Design review of the part built by this model. Coordinates are the model's own, in mm. Coordinates: 2 decimals unless noted, no trailing zeros. Write each loop counter-clockwise with the first axis right and the second up, starting at its lowest first coordinate (ties: lowest second). Pieces come first, ordered by that corner, then holes.
Q1. Take a section at A-A (z = 11.5). Give the boundary of the cut face in (x, y) (3 decimals), and give its area (3 significant figures).
Q2. Mouldability with a two-part tool opening along X and no side actions: class faces 1 (the cylindrical face through (30.229, 1.493, -18.726)), 2 (the cylindrical face through (-16.854, 1.479, -12.63)), 3 (the flat face through (3, 3, 2)) as pulls with the +X half, pulls with the -X half, needs draft (parallel to the pull), parting line crosses it, or undercut.
Q3. For probe 1 along X at (y, z) = (1.8, 11.5) (3 decimals); probe 2 along X at (y, z) = (1.7, -12.5) (3 decimals); probe 3 along X at (y, z) = (2.3, 11.5) (3 decimals), list the stretches that pass through material, from the lowest coordinate up.
Q4. Take a section at B-B (z = -12.5). Give the boundary of the cut face in (x, y) (3 decimals).
```python
from build123d import *

# Parameters (mm, degrees)
SKETCH1_R           = 1
BOSS_EXTRUDE1_DEPTH = 3
FILLET1_R           = 1


with BuildPart() as part:
    # Sketch1 → Boss-Extrude1 (new body)
    with BuildSketch(Plane(origin=(0, 0, 0), x_dir=(-1, 0, 0), z_dir=(0, 1, 0))):
        with BuildLine():
            Line((-31.655, 18.23), (-31.655, -15.23))
            ThreePointArc((-31.655, -15.23), (-30.190533906, -18.765533906), (-26.655, -20.23))
            Line((-26.655, -20.23), (20.655, -20.23))
            ThreePointArc((20.655, -20.23), (24.190533906, -18.765533906), (25.655, -15.23))
            Line((25.655, -15.23), (25.655, 18.23))
            ThreePointArc((25.655, 18.23), (24.190533906, 21.765533906), (20.655, 23.23))
            Line((20.655, 23.23), (-26.655, 23.23))
            ThreePointArc((-26.655, 23.23), (-30.190533906, 21.765533906), (-31.655, 18.23))
        make_face()
        with Locations(Location((-18.155, 11.5, 0), (0, 0, 90))):
            Circle(SKETCH1_R, mode=Mode.SUBTRACT)
        with Locations(Location((17.845, 11.5, 0), (0, 0, 90))):
            Circle(SKETCH1_R, mode=Mode.SUBTRACT)
        with Locations(Location((17.845, -12.5, 0), (0, 0, 90))):
            Circle(SKETCH1_R, mode=Mode.SUBTRACT)
    extrude(amount=BOSS_EXTRUDE1_DEPTH)

    # Fillet1
    fillet1_edges = [part.edges().sort_by_distance(p)[0] for p in [
        (30.190533906, 3, -18.765533906),
        (31.655, 0, 1.5),
        (30.190533906, 0, 21.765533906),
        (3, 3, -20.23),
        (-24.190533906, 3, -18.765533906),
        (-25.655, 3, 1.5),
        (-24.190533906, 3, 21.765533906),
        (3, 3, 23.23),
        (30.190533906, 3, 21.765533906),
        (31.655, 3, 1.5),
        (3, 0, 23.23),
        (-24.190533906, 0, 21.765533906),
        (-25.655, 0, 1.5),
        (-24.190533906, 0, -18.765533906),
        (3, 0, -20.23),
        (30.190533906, 0, -18.765533906),
    ]]
    fillet(fillet1_edges, radius=FILLET1_R)


solid = part.part
```
Response:
1. outline: (-25.655, 1) arc R1 ccw to (-24.655, 0) - (-18.845, 0) - (-18.845, 3) - (-24.655, 3) arc R1 ccw to (-25.655, 2) - close; (-16.845, 0) - (17.155, 0) - (17.155, 3) - (-16.845, 3) - close; (19.155, 0) - (30.655, 0) arc R1 ccw to (31.655, 1) - (31.655, 2) arc R1 ccw to (30.655, 3) - (19.155, 3) - close
1. area: 159 mm2
2. face 1: pulls with the +X half
2. face 2: undercut
2. face 3: needs draft
3. probe 1: x = -25.655 to -18.845, -16.845 to 17.155, 19.155 to 31.655
3. probe 2: x = -25.655 to -18.845, -16.845 to 31.655
3. probe 3: x = -25.609 to -18.845, -16.845 to 17.155, 19.155 to 31.609
4. outline: (-25.655, 1) arc R1 ccw to (-24.655, 0) - (-18.845, 0) - (-18.845, 3) - (-24.655, 3) arc R1 ccw to (-25.655, 2) - close; (-16.845, 0) - (30.655, 0) arc R1 ccw to (31.655, 1) - (31.655, 2) arc R1 ccw to (30.655, 3) - (-16.845, 3) - close
